```python
from build123d import *

# Parameters (mm, degrees)
BOSS_EXTRUDE1_DEPTH = 5
FILLET1_R           = 1


with BuildPart() as part:
    # Sketch2 → Boss-Extrude1 (new, symmetric)
    with BuildSketch(Plane.XY):
        with BuildLine():
            Line((-6, 0), (-6, 20))
            Line((-6, 20), (6, 20))
            Line((6, 20), (6, 0))
            ThreePointArc((6, 0), (0, -6), (-6, 0))
        make_face()
    extrude(amount=BOSS_EXTRUDE1_DEPTH, both=True)

    # Fillet1
    fillet1_edges = [part.edges().sort_by_distance(p)[0] for p in [
        (-6, 10, 5),
        (0, -6, 5),
        (-6, 10, -5),
        (6, 10, -5),
        (0, -6, -5),
        (6, 10, 5),
    ]]
    fillet(fillet1_edges, radius=FILLET1_R)


solid = part.part
```
Check sheet for the modelled part. Datum: model origin and axes. Units: mm. Round coordinates to 2 decimals unless told otherwise and drop trailing zeros. Order: outer loops, then holes, each group sorted by start corner. A loop starts at its lowest first (then second) coordinate and runs counter-clockwise, first axis right, second up. Notation, with made-up numbers: M -26,32 L -6,32 A24 cw -6,68 Z; hole C 12,10 d7. An arc over 180 degrees is marked long. Answer in a Markdown table with one row per item.
(1) Material ranges on line 1 along X through (y, z) = (-3, -3); line 2 along Y through (x, z) = (-1, 1); line 3 along Y through (x, z) = (3.5, -1.75), recorded low to high. Write a range as from..to.
Findings:
| item | result |
|---|---|
| line 1 | x = -5.2..5.2 |
| line 2 | y = -5.92..20 |
| line 3 | y = -4.87..20 |
(2) Gauge pin test, flat ends, axial feed: pin 1 (1 mm diameter, centred on x = -1, z = -2, fed in from -Y); pin 2 (1.5 mm diameter, centred on x = -2, z = -3, fed in from -Y). Record the tip position at first contact, or that the pin passes through.
Findings:
| item | result |
|---|---|
| pin 1 | stops at y = -5.98 |
| pin 2 | stops at y = -5.87 |
(3) Section check A-A on z = 3. Record the boundary of the cut face in (x, y), plus the area to 3 significant figures.
Findings:
| item | result |
|---|---|
| outline | M -6,0 A6 ccw 6,0 L 6,20 L -6,20 Z |
| area | 297 mm^2 |
